```python
from build123d import *

# Parameters (mm, degrees)
SKETCH_1_R          = 3.95
EXTRUDE_1_DEPTH     = 4
EXTRUDE_1_TAPER     = 7.5
SKETCH_2_R          = 1.5
CUT_EXTRUDE_1_DEPTH = 4
EXTRUDE_2_DEPTH     = 0.5


with BuildPart() as part:
    # 草图1 → 凸台-拉伸1 (new body)
    with BuildSketch(Plane(origin=(0, 0, 0), x_dir=(1, 0, 0), z_dir=(0, 1, 0))):
        Circle(SKETCH_1_R)
    extrude(amount=EXTRUDE_1_DEPTH, taper=EXTRUDE_1_TAPER)

    # 草图2 → 切除-拉伸1 (cut)
    with BuildSketch(Plane(origin=(0, 0, 0), x_dir=(1, 0, 0), z_dir=(0, 1, 0))):
        Circle(SKETCH_2_R)
    extrude(amount=CUT_EXTRUDE_1_DEPTH, mode=Mode.SUBTRACT)

    # 草图3 → 凸台-拉伸2 (add, symmetric)
    with BuildSketch(Plane.XY):
        with BuildLine():
            Line((8.380151519, 4.430151519), (3.95, 0))
            Line((3.95, 0), (1.95, 0))
            Line((1.95, 0), (1.95, 4))
            Line((1.95, 4), (3.42339001, 4))
            Line((3.42339001, 4), (3.907794349, 7.679416256))
            ThreePointArc((3.907794349, 7.679416256), (4.291558837, 8.619529341), (5.087532952, 9.250015662))
            ThreePointArc((5.087532952, 9.250015662), (8.73241738, 8.205380502), (8.380151519, 4.430151519))
        make_face()
        with BuildLine():
            Line((-1.95, 4), (-1.95, 0))
            Line((-1.95, 0), (-3.95, 0))
            Line((-3.95, 0), (-8.380151519, 4.430151519))
            ThreePointArc((-8.380151519, 4.430151519), (-8.73241738, 8.205380502), (-5.087532952, 9.250015662))
            ThreePointArc((-5.087532952, 9.250015662), (-4.291558837, 8.619529341), (-3.907794349, 7.679416256))
            Line((-3.907794349, 7.679416256), (-3.42339001, 4))
            Line((-3.42339001, 4), (-1.95, 4))
        make_face()
    extrude(amount=EXTRUDE_2_DEPTH, both=True)


solid = part.part
```
CAD build for the part. Positions are in the model's coordinates, mm. A direction names the side the tool comes from. Round coordinates to 2 decimals unless told otherwise and drop trailing zeros. Write each loop counter-clockwise with the first axis right and the second up, starting at its lowest first coordinate (ties: lowest second). Pieces come first, ordered by that corner, then holes.
Item 1: Band-saw the part on D-D on y = 0.75. Write the cut outline in (x, z).
Filled in:
outline: (-4.7, -0.5) - (-3.82, -0.5) arc R3.85 ccw to (3.82, -0.5) - (4.7, -0.5) - (4.7, 0.5) - (3.82, 0.5) arc R3.85 ccw to (-3.82, 0.5) - (-4.7, 0.5) - close; hole circle Ø3 at (0, 0)
Item 2: Drill centre lines: L1, parallel to Z at x = 0, y = 2.7; L2, parallel to Z at x = -6.5, y = 6.25; L3, parallel to X at y = 2.55, z = 0. Where is each one in solid material? Low to high.
Filled in:
L1: z = -3.59 to -1.5, 1.5 to 3.59
L2: z = -0.5 to 0.5
L3: x = -6.5 to -1.5, 1.5 to 6.5
Item 3: Band-saw the part on A-A on x = 0. Write the cut outline in (y, z), then the cut area to 3 significant figures.
Filled in:
outline: (0, -3.95) - (4, -3.42) - (4, -1.5) - (0, -1.5) - close; (0, 1.5) - (4, 1.5) - (4, 3.42) - (0, 3.95) - close
area: 17.5 mm2
Item 4: Tool access for faces 5 (the cylindrical face through (-4.3, 8.63, 0.01)), 6 (the conical face through (0.074, 2.028, -3.682)): list every direction of +Z, -Z, +X, -X, +Y, -Y with a clear straight run to the whole face (end or side of a thin tool).
Filled in:
face 5: +Z, -Z, +Y
face 6: -Z, +Y
Item 5: Mould opens along X. For faces 1 (the flat face through (-6.13, 2.18, 0.01)), 2 (the cylindrical face through (4.283, 8.608, -0.007)), 3 (the flat face through (-2, 0, 0)), 4 (the conical face through (-0.074, 2.028, 3.682)) say: released by +X, released by -X, zero draft, split by the parting line, or undercut.
Filled in:
face 1: released by -X
face 2: undercut
face 3: zero draft
face 4: split by the parting line
Item 6: Band-saw the part on B-B on y = 5.5. Write the cut outline in (x, z), then the cut area to 3 significant figures.
Filled in:
outline: (-9.07, -0.5) - (-3.62, -0.5) - (-3.62, 0.5) - (-9.07, 0.5) - close; (3.62, -0.5) - (9.07, -0.5) - (9.07, 0.5) - (3.62, 0.5) - close
area: 10.9 mm2
Item 7: Drop flat-ended pins along their axis: pin 1 Ø1.8 at (x, y) = (-7.5, 4.5) entering from +Z; pin 2 Ø5 at (x, y) = (2, 3.5) entering from -Z; pin 3 Ø1.8 at (x, y) = (6.5, 3.5) entering from -Z. Give the stop position or say it passes through.
Filled in:
pin 1: stops at z = 0.5
pin 2: stops at z = -3.72
pin 3: stops at z = -0.5
Item 8: Band-saw the part on C-C on z = 0. Write the cut outline in (x, y).
Filled in:
outline: (-8.38, 4.43) - (-3.95, 0) - (-1.5, 0) - (-1.5, 4) - (-3.42, 4) - (-3.91, 7.68) arc R2 ccw to (-5.09, 9.25) arc R2.97 ccw to start; (1.5, 0) - (3.95, 0) - (8.38, 4.43) arc R2.97 ccw to (5.09, 9.25) arc R2 ccw to (3.91, 7.68) - (3.42, 4) - (1.5, 4) - close
